For this review, take the finished solid that the model builds, in its own axes (mm). A direction names the side the tool comes from. Coordinates: 2 decimals unless noted, no trailing zeros. Loops run counter-clockwise (first coordinate to the right, second up) from the corner with the lowest first, then second, coordinate; pieces in that order, holes last. Notation, with made-up numbers: M 81,72 L 118,72 A19 ccw 118,77 Z; hole C 29.5,40 d9. An arc over 180 degrees is marked long. Use one line per item in the form item = value.
```python
from build123d import *

# Parameters (mm, degrees)
SKETCH2_W = 2.5
SKETCH2_H = 2.5


with BuildPart() as part:
    # Sketch1 → Revolve1 (revolve)
    with BuildSketch(Plane.XY, mode=Mode.PRIVATE) as revolve1_sk:
        Polygon((0, 0), (5, 0), (5, -23), (6.25, -23), (6.25, -28), (0, -28), align=None)
    revolve(revolve1_sk.sketch.rotate(Axis((0, 5, 0), (0, -1, 0)), 180), axis=Axis((0, 5, 0), (0, -1, 0)))

    # Sketch2 → Cut-Revolve1 (revolve, cut)
    with BuildSketch(Plane.XY, mode=Mode.PRIVATE) as cut_revolve1_sk:
        with Locations((3.75, -3.75)):
            Rectangle(SKETCH2_W, SKETCH2_H)
    revolve(cut_revolve1_sk.sketch.rotate(Axis((0, 0, 0), (0, -1, 0)), 180), axis=Axis((0, 0, 0), (0, -1, 0)), mode=Mode.SUBTRACT)


solid = part.part
```
1. Draft analysis for pull direction Y (two halves, no side actions). For faces 1 (the face through (0, -28, 0)), 2 (the face through (2, -2.5, 2)), 3 (the face through (-5.96, -25.54, -1.88)), state which applies: +Y half, -Y half, draft (parallel to the pull), parting line (faces both ways), or undercut.
Computed values:
face_1 = -Y half
face_2 = undercut
face_3 = draft
2. Consider section D-D on z = 0. Write out the cut boundary in (x, y), plus the area to 3 significant figures.
Computed values:
outline = M -6.25,-28 L 6.25,-28 L 6.25,-23 L 5,-23 L 5,-5 L 2.5,-5 L 2.5,-2.5 L 5,-2.5 L 5,0 L -5,0 L -5,-2.5 L -2.5,-2.5 L -2.5,-5 L -5,-5 L -5,-23 L -6.25,-23 Z
area = 280 mm2
3. For pin 1 Ø1 at (x, y) = (2, -15.5) entering from +Z; pin 2 Ø2 at (x, y) = (-1, -19) entering from +Z; pin 3 Ø1 at (x, y) = (-4.5, -13) entering from -Z, all flat-tipped, find the tip position at first contact; note any pin that passes through.
Computed values:
pin_1 = 4.77
pin_2 = 5
pin_3 = -3
4. Consider section A-A on x = 0. Write out the cut boundary in (y, z), plus the area to 3 significant figures.
Computed values:
outline = M -28,-6.25 L -23,-6.25 L -23,-5 L -5,-5 L -5,-2.5 L -2.5,-2.5 L -2.5,-5 L 0,-5 L 0,5 L -2.5,5 L -2.5,2.5 L -5,2.5 L -5,5 L -23,5 L -23,6.25 L -28,6.25 Z
area = 280 mm2
5. Consider section C-C on x = -3.5. Write out the cut boundary in (y, z), plus the area to 3 significant figures.
Computed values:
outline = M -28,-5.18 L -23,-5.18 L -23,-3.57 L -5,-3.57 L -5,3.57 L -23,3.57 L -23,5.18 L -28,5.18 Z; M -2.5,-3.57 L 0,-3.57 L 0,3.57 L -2.5,3.57 Z
area = 198 mm2
6. Wall thickness on line 1 along Y through (x, z) = (4.25, 0.5); line 2 along Z through (x, y) = (0, -20.75); line 3 along Z through (x, y) = (-2.25, -24.25): over which ranges is each line inside the solid? List them lowest first. Write a range as from..to.
Computed values:
line_1 = -28..-5, -2.5..0
line_2 = -5..5
line_3 = -5.83..5.83
7. Consider section B-B on z = -4.5. Write out the cut boundary in (x, y), plus the area to 3 significant figures.
Computed values:
outline = M -4.34,-28 L 4.34,-28 L 4.34,-23 L 2.18,-23 L 2.18,-5 L -2.18,-5 L -2.18,-23 L -4.34,-23 Z; M -2.18,-2.5 L 2.18,-2.5 L 2.18,0 L -2.18,0 Z
area = 133 mm2
8. Tool access review of faces 4 (the face through (0, 0, 0)), 5 (the face through (2, -23, -5)), 6 (the face through (2, -5, 2)): name each direction out of +Z, -Z, +X, -X, +Y, -Y from which nothing blocks a thin tool from reaching the whole face with its end or side.
Computed values:
face_4 = +Z, -Z, +X, -X, +Y
face_5 = +Y
face_6 = none
